```python
from build123d import *

# Parameters (mm, degrees)
SKETCH1_R           = 2.55
BOSS_EXTRUDE1_DEPTH = 3
SKETCH2_R           = 1.55
GIMBALHOLES_DEPTH   = 3
FILLET1_R           = 10
FILLET2_R           = 5


with BuildPart() as part:
    # Sketch1 → Boss-Extrude1 (new body)
    with BuildSketch(Plane(origin=(0, 0, 0), x_dir=(1, 0, 0), z_dir=(0, 1, 0))):
        with BuildLine():
            Line((-60, 27.5), (-60, -27.5))
            ThreePointArc((-60, -27.5), (-70, -37.5), (-60, -47.5))
            Line((-60, -47.5), (-60, -98.5))
            Line((-60, -98.5), (60.000001096, -98.5))
            Line((60.000001096, -98.5), (60.000001096, -47.5))
            ThreePointArc((60.000001096, -47.5), (70, -37.499999452), (60, -27.5))
            Line((60, -27.5), (60, 27.5))
            ThreePointArc((60, 27.5), (70, 37.499999452), (60.000001096, 47.5))
            Line((60.000001096, 47.5), (60.000001096, 98.5))
            Line((60.000001096, 98.5), (-60, 98.5))
            Line((-60, 98.5), (-60, 47.5))
            ThreePointArc((-60, 47.5), (-70, 37.5), (-60, 27.5))
        make_face()
        with Locations(Location((-60, 37.5, 0), (0, 0, 270))):
            Circle(SKETCH1_R, mode=Mode.SUBTRACT)
        with Locations(Location((60, 37.5, 0), (0, 0, 270))):
            Circle(SKETCH1_R, mode=Mode.SUBTRACT)
        with Locations(Location((-60, -37.5, 0), (0, 0, 270))):
            Circle(SKETCH1_R, mode=Mode.SUBTRACT)
        with Locations(Location((60, -37.5, 0), (0, 0, 270))):
            Circle(SKETCH1_R, mode=Mode.SUBTRACT)
    extrude(amount=BOSS_EXTRUDE1_DEPTH)

    # Sketch2 → GimbalHoles (cut)
    with BuildSketch(Plane(origin=(0, 3, 0), x_dir=(1, 0, 0), z_dir=(0, 1, 0))):
        with Locations(Location((-44.999998904, 73.5, 0), (0, 0, 270))):
            Circle(SKETCH2_R)
        with Locations(Location((-24.999998904, 73.5, 0), (0, 0, 270))):
            Circle(SKETCH2_R)
        with Locations(Location((25.000001096, 73.5, 0), (0, 0, 270))):
            Circle(SKETCH2_R)
        with Locations(Location((45.000001096, 73.5, 0), (0, 0, 270))):
            Circle(SKETCH2_R)
        with Locations(Location((-44.999998904, -73.5, 0), (0, 0, 270))):
            Circle(SKETCH2_R)
        with Locations(Location((-24.999998904, -73.5, 0), (0, 0, 270))):
            Circle(SKETCH2_R)
        with Locations(Location((25.000001096, -73.5, 0), (0, 0, 270))):
            Circle(SKETCH2_R)
        with Locations(Location((45.000001096, -73.5, 0), (0, 0, 270))):
            Circle(SKETCH2_R)
    extrude(amount=-GIMBALHOLES_DEPTH, mode=Mode.SUBTRACT)

    # Fillet1
    fillet1_edges = [part.edges().sort_by_distance(p)[0] for p in [
        (-60, 1.5, -98.5),
        (60.000001096, 1.5, -98.5),
        (60.000001096, 1.5, 98.5),
        (-60, 1.5, 98.5),
    ]]
    fillet(fillet1_edges, radius=FILLET1_R)

    # Fillet2
    fillet2_edges = [part.edges().sort_by_distance(p)[0] for p in [
        (-60, 1.5, -47.5),
        (60.000001096, 1.5, -47.5),
        (60, 1.5, -27.5),
        (60, 1.5, 27.5),
        (60.000001096, 1.5, 47.5),
        (-60, 1.5, 47.5),
        (-60, 1.5, 27.5),
        (-60, 1.5, -27.5),
    ]]
    fillet(fillet2_edges, radius=FILLET2_R)


solid = part.part
```
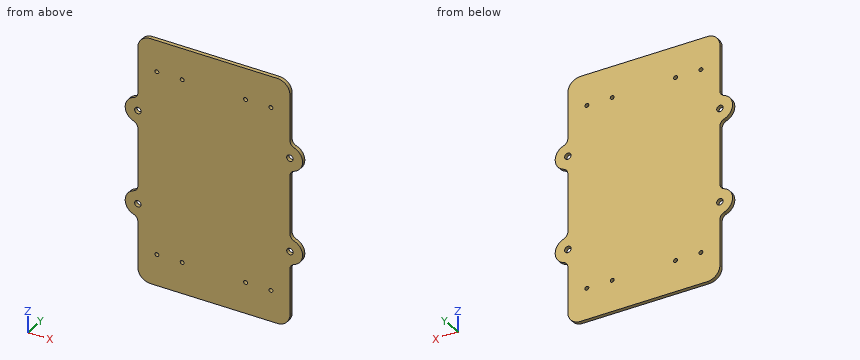
Can you work these out from the model? Positions are in its coordinate system, mm. Coordinates: 2 decimals unless noted, no trailing zeros. Order: outer loops, then holes, each group sorted by start corner. A loop starts at its lowest first (then second) coordinate and runs counter-clockwise, first axis right, second up.
1. I'm going to push flat-ended pins straight in: pin 1 (0.9 mm diameter, centred on y = 1.5, z = 3, fed in from +X); pin 2 (1.5 mm diameter, centred on y = 1.5, z = -71.5, fed in from -X); pin 3 (1.5 mm diameter, centred on y = 2.5, z = -47.5, fed in from +X). Where does each tip first touch, or does it pass through?
2. I need wall thicknesses on line 1 (X direction, y = 1.4, z = -37.5); line 2 (X direction, y = 2.35, z = 73.5); line 3 (Z direction, x = -24.5, y = 2.25). Which ranges of each line are inside material? Lowest first, please.
3. If we section it at C-C (y = 2.1): Give the number of separate pieces and of enclosed holes in the cut face, then the cut area to 3 significant figures.
4. If we section it at A-A (z = 37.5): Please give me the cut outline in (x, y).
5. If we section it at B-B (z = 15.5): Please give me the cut outline in (x, y), then the cut area to 3 significant figures.
Entries:
1. pin 1: stops at x = 60
1. pin 2: stops at x = -60
1. pin 3: stops at x = 63.8
2. line 1: x = -70 to -62.55, -57.45 to 57.45, 62.55 to 70
2. line 2: x = -60 to -46.55, -43.45 to -26.55, -23.45 to 23.45, 26.55 to 43.45, 46.55 to 60
2. line 3: z = -98.5 to -74.97, -72.03 to 72.03, 74.97 to 98.5
3. separate pieces: 1
3. enclosed holes: 12
3. area: 24,100 mm2
4. outline: (-70, 0) - (-62.55, 0) - (-62.55, 3) - (-70, 3) - close; (-57.45, 0) - (57.45, 0) - (57.45, 3) - (-57.45, 3) - close; (62.55, 0) - (70, 0) - (70, 3) - (62.55, 3) - close
5. outline: (-60, 0) - (60, 0) - (60, 3) - (-60, 3) - close
5. area: 360 mm2
